Source: CAD feature listing. Evaluate the final solid. Frame: model axes, mm. Round coordinates to 2 decimals unless told otherwise and drop trailing zeros. Write each loop counter-clockwise with the first axis right and the second up, starting at its lowest first coordinate (ties: lowest second). Pieces come first, ordered by that corner, then holes. Notation, with made-up numbers: M 70.25,1 L 93.25,1 A25 cw 93.25,16 Z; hole C 87,-35 d5. An arc over 180 degrees is marked long. Answer in a Markdown table with one row per item.
from build123d import *
from build123d.topology import SkipClean

# Parameters (mm, degrees)
CROQUIS1_R                                           = 25
SALIENTE_EXTRUIR1_DEPTH                              = 5
CROQUIS2_R                                           = 2.7
CORTAR_EXTRUIR2_DEPTH                                = 5
CROQUIS3_R                                           = 1.45
CORTAR_EXTRUIR3_DEPTH                                = 5
CROQUIS4_R                                           = 10.6
CORTAR_EXTRUIR4_DEPTH                                = 5
CORTAR_EXTRUIR4_DRAFT                                = -1.5
AVELLANADO_PARA_TORNILLO_CON_CABEZA_PLAN_D           = 3.6
AVELLANADO_PARA_TORNILLO_CON_CABEZA_PLAN_CSINK_D     = 6.3
AVELLANADO_PARA_TORNILLO_CON_CABEZA_PLAN_CSINK_ANGLE = 90
CROQUIS7_R                                           = 2.7
SALIENTE_EXTRUIR2_DEPTH                              = 1
REDONDEO1_R                                          = 1


with BuildPart() as part:
    # Croquis1 → Saliente-Extruir1 (new body)
    with BuildSketch(Plane(origin=(0, 0, 0), x_dir=(1, 0, 0), z_dir=(0, 1, 0))):
        with Locations(Location((0, 0, 0), (0, 0, 270))):
            Circle(CROQUIS1_R)
    extrude(amount=SALIENTE_EXTRUIR1_DEPTH)

    # Croquis2 → Cortar-Extruir2 (cut)
    with BuildSketch(Plane(origin=(0, 5, 0), x_dir=(1, 0, 0), z_dir=(0, 1, 0))):
        with Locations(Location((0, 21.42, 0), (0, 0, 270))):
            Circle(CROQUIS2_R)
        with Locations(Location((18.550264149, -10.71, 0), (0, 0, 270))):
            Circle(CROQUIS2_R)
        with Locations(Location((-18.550264149, -10.71, 0), (0, 0, 270))):
            Circle(CROQUIS2_R)
    extrude(amount=-CORTAR_EXTRUIR2_DEPTH, mode=Mode.SUBTRACT)

    # Croquis3 → Cortar-Extruir3 (cut)
    with BuildSketch(Plane(origin=(0, 5, 0), x_dir=(1, 0, 0), z_dir=(0, 1, 0))):
        with Locations(Location((0, -21.5, 0), (0, 0, 270))):
            Circle(CROQUIS3_R)
        with Locations(Location((-18.619546181, 10.75, 0), (0, 0, 270))):
            Circle(CROQUIS3_R)
        with Locations(Location((18.619546181, 10.75, 0), (0, 0, 270))):
            Circle(CROQUIS3_R)
    extrude(amount=-CORTAR_EXTRUIR3_DEPTH, mode=Mode.SUBTRACT)


with BuildPart() as cortar_extruir4_tool:
    # Croquis4 → Cortar-Extruir4 (with draft: the straight prism first)
    with BuildSketch(Plane(origin=(0, 5, 0), x_dir=(1, 0, 0), z_dir=(0, 1, 0))):
        Circle(CROQUIS4_R)
    extrude(amount=-CORTAR_EXTRUIR4_DEPTH)
    # Cortar-Extruir4: the draft: its side faces are tilted about the plane it starts from
    cortar_extruir4_sides = [cortar_extruir4_tool.faces().sort_by_distance(p)[0] for p in [
        (-10.6, 2.5, 0),
    ]]
    draft(cortar_extruir4_sides, Plane(origin=(0, 5, 0), x_dir=(1, 0, 0), z_dir=(0, 1, 0)), CORTAR_EXTRUIR4_DRAFT)


with BuildPart() as part_1:
    add(part.part)

    # Cortar-Extruir4: cut by cortar_extruir4_tool
    add(cortar_extruir4_tool.part, mode=Mode.SUBTRACT)

    # Avellanado para tornillo con cabeza plana de M31 (through all)
    with Locations(Plane(origin=(0, 5, 0), x_dir=(1, 0, 0), z_dir=(0, 1, 0))):
        with Locations((-18.619546181, 10.75), (18.619546181, 10.75), (0, -21.5)):
            CounterSinkHole(AVELLANADO_PARA_TORNILLO_CON_CABEZA_PLAN_D / 2, AVELLANADO_PARA_TORNILLO_CON_CABEZA_PLAN_CSINK_D / 2, counter_sink_angle=AVELLANADO_PARA_TORNILLO_CON_CABEZA_PLAN_CSINK_ANGLE)

    # Croquis7 → Saliente-Extruir2 (add)
    # profile 1 of 3: a face of its own
    with SkipClean():  # the faces are left unmerged after this step: merging them gives an invalid solid
        with BuildSketch(Plane(origin=(0, 0, 0), x_dir=(-1, 0, 0), z_dir=(0, -1, 0))):
            with BuildLine():
                ThreePointArc((22.549366787, -10.794723595), (15.086162534, -8.71), (20.623188254, -14.13096268))
                ThreePointArc((20.623188254, -14.13096268), (21.650635095, -12.5), (22.549366787, -10.794723595))
            make_face()
            with Locations(Location((18.550264149, -10.71, 0), (0, 0, 270))):
                Circle(CROQUIS7_R, mode=Mode.SUBTRACT)
        # profile 2 of 3: a face of its own
        with BuildSketch(Plane(origin=(0, 0, 0), x_dir=(-1, 0, 0), z_dir=(0, -1, 0))):
            with BuildLine():
                ThreePointArc((-20.623188254, -14.13096268), (-15.086162534, -8.71), (-22.549366787, -10.794723595))
                ThreePointArc((-22.549366787, -10.794723595), (-21.650635095, -12.5), (-20.623188254, -14.13096268))
            make_face()
            with Locations(Location((-18.550264149, -10.71, 0), (0, 0, 270))):
                Circle(CROQUIS7_R, mode=Mode.SUBTRACT)
        # profile 3 of 3: a face of its own
        with BuildSketch(Plane(origin=(0, 0, 0), x_dir=(-1, 0, 0), z_dir=(0, -1, 0))):
            with BuildLine():
                ThreePointArc((-1.926178534, 24.925686275), (0, 17.42), (1.926178534, 24.925686275))
                ThreePointArc((1.926178534, 24.925686275), (0, 25), (-1.926178534, 24.925686275))
            make_face()
            with Locations(Location((0, 21.42, 0), (0, 0, 270))):
                Circle(CROQUIS7_R, mode=Mode.SUBTRACT)
        extrude(amount=SALIENTE_EXTRUIR2_DEPTH)

    # Redondeo1
    # the kernel refuses this fillet: 1 mm, written as the material it adds along each edge
    with BuildSketch(Plane(origin=(0, 0, -21.42), x_dir=(0.0031415874858800596, 0, -0.9999950652018583), z_dir=(-0.9999950652018583, 0, -0.0031415874858800596))) as redondeo1_piece_1_section:
        with BuildLine():
            CenterArc((4 + REDONDEO1_R, REDONDEO1_R), REDONDEO1_R, 180, 90)
            Line((4, REDONDEO1_R), (4, 0))
            Line((4, 0), (4 + REDONDEO1_R, 0))
        make_face()
    redondeo1_piece_1 = revolve(axis=Axis((0, 0, -21.42), (0, -1, 0)), revolution_arc=359.64, mode=Mode.PRIVATE)
    redondeo1_piece_1 = redondeo1_piece_1 & Plane(origin=(0, -0.280437839, 0), x_dir=(0, 0, 1), z_dir=(0, -1, 0)) * Cylinder(25, 21, mode=Mode.PRIVATE)
    add(redondeo1_piece_1)
    with BuildSketch(Plane(origin=(18.550264149, 0, 10.71), x_dir=(0.8644503363809782, 0, 0.5027182271718559), z_dir=(0.5027182271718559, 0, -0.8644503363809782))) as redondeo1_piece_2_section:
        with BuildLine():
            CenterArc((4 + REDONDEO1_R, REDONDEO1_R), REDONDEO1_R, 180, 90)
            Line((4, REDONDEO1_R), (4, 0))
            Line((4, 0), (4 + REDONDEO1_R, 0))
        make_face()
    redondeo1_piece_2 = revolve(axis=Axis((18.550264149, 0, 10.71), (0, -1, 0)), revolution_arc=359.64, mode=Mode.PRIVATE)
    redondeo1_piece_2 = redondeo1_piece_2 & Plane(origin=(0, -0.280437839, 0), x_dir=(0, 0, 1), z_dir=(0, -1, 0)) * Cylinder(25, 21, mode=Mode.PRIVATE)
    add(redondeo1_piece_2)
    with BuildSketch(Plane(origin=(-18.550264149, 0, 10.71), x_dir=(-0.867591923866794, 0, 0.49727683803000045), z_dir=(0.49727683803000045, 0, 0.867591923866794))) as redondeo1_piece_3_section:
        with BuildLine():
            CenterArc((4 + REDONDEO1_R, REDONDEO1_R), REDONDEO1_R, 180, 90)
            Line((4, REDONDEO1_R), (4, 0))
            Line((4, 0), (4 + REDONDEO1_R, 0))
        make_face()
    redondeo1_piece_3 = revolve(axis=Axis((-18.550264149, 0, 10.71), (0, -1, 0)), revolution_arc=359.64, mode=Mode.PRIVATE)
    redondeo1_piece_3 = redondeo1_piece_3 & Plane(origin=(0, -0.280437839, 0), x_dir=(0, 0, 1), z_dir=(0, -1, 0)) * Cylinder(25, 20, mode=Mode.PRIVATE)
    add(redondeo1_piece_3)


solid = part_1.part
Q1. Section D-D (z = -21.42). Return loops of the section in (x, y), and give its area (3 significant figures).
Solutions:
| item | result |
|---|---|
| outline | M -12.89,0 L -5,0 A1 cw -4,-1 L -2.7,-1 L -2.7,5 L -12.89,5 Z; M 2.7,-1 L 4,-1 A1 cw 5,0 L 12.89,0 L 12.89,5 L 2.7,5 Z |
| area | 105 mm2 |
Q2. Section B-B (y = 2.75). Return loops of the section in (x, z), and give its area (3 significant figures).
Solutions:
| item | result |
|---|---|
| outline | C 0,0 d50; hole C -18.55,10.71 d5.4; hole C -18.62,-10.75 d3.6; hole C 0,0 d21.08; hole C 0,-21.42 d5.4; hole C 0,21.5 d3.6; hole C 18.55,10.71 d5.4; hole C 18.62,-10.75 d3.6 |
| area | 1,520 mm2 |
Q3. Contact query for flat-ended pins moving along their axis: pin 1 Ø6 at (x, z) = (0, 21.5) entering from -Y; pin 2 Ø4 at (x, z) = (18.62, -10.75) entering from +Y; pin 3 Ø3 at (x, y) = (-6.5, 1.5) entering from -Z. Output: stop coordinate, or through.
Solutions:
| item | result |
|---|---|
| pin 1 | stops at y = 0 |
| pin 2 | stops at y = 3.85 |
| pin 3 | stops at z = -24.49 |
Q4. Section C-C (x = 0). Return loops of the section in (y, z), and give its area (3 significant figures).
Solutions:
| item | result |
|---|---|
| outline | M -1,-25 L 5,-25 L 5,-24.12 L -1,-24.12 Z; M -1,-18.72 L 5,-18.72 L 5,-10.6 L 0,-10.47 L 0,-16.42 A1 cw -1,-17.42 Z; M 0,10.47 L 5,10.6 L 5,18.35 L 3.65,19.7 L 0,19.7 Z; M 0,23.3 L 3.65,23.3 L 5,24.65 L 5,25 L 0,25 Z |
| area | 100 mm2 |
Q5. Pull-direction query (X, two-part tool) for faces 1 (the flat face through (-11, 5, 0)), 2 (the cylindrical face through (-20.3, 1.8, -10.1)), 3 (the conical face through (-8.36, 2.53, 6.41)); classes: pulls with the +X half, pulls with the -X half, needs draft (parallel to the pull), parting line crosses it, or undercut.
Solutions:
| item | result |
|---|---|
| face 1 | needs draft |
| face 2 | undercut |
| face 3 | undercut |
Q6. Material intervals for probe 1 along X at (y, z) = (4, 8.5); probe 2 along Z at (x, y) = (1.5, 2.5) (3 decimals); probe 3 along Z at (x, y) = (7, 3.5), sorted ascending.
Solutions:
| item | result |
|---|---|
| probe 1 | x = -23.51 to -20.1, -17 to -6.29, 6.29 to 17, 20.1 to 23.51 |
| probe 2 | z = -24.955 to -23.665, -19.175 to -10.427, 10.427 to 20.505, 22.495 to 24.955 |
| probe 3 | z = -24 to -7.91, 7.91 to 24 |
Q7. Section A-A (z = 0). Return loops of the section in (x, y), and give its area (3 significant figures).
Solutions:
| item | result |
|---|---|
| outline | M -25,0 L -10.47,0 L -10.6,5 L -25,5 Z; M 10.47,0 L 25,0 L 25,5 L 10.6,5 Z |
| area | 145 mm2 |
